from build123d import *

# Parameters (mm, degrees)
PAD005_DEPTH = 9.8
SKETCH007_R  = 6.5
PAD006_DEPTH = 9.8
PAD004_DEPTH = 9.8


with BuildPart() as pad005:
    # Sketch005 → Pad005 (new body)
    with BuildSketch(Plane.XZ.offset(-5)):
        with BuildLine():
            ThreePointArc((42.504006, 47.762261), (40.661796, 52.159127), (36.195109, 53.824922))
            ThreePointArc((23.79127, 66.581039), (27.163695, 57.451626), (36.195109, 53.824922))
            Line((23.79127, 66.581039), (23.79127, 71.581039))
            Line((23.79127, 71.581039), (29.771593, 65.581039))
            ThreePointArc((29.771593, 65.581039), (31.67487, 61.429233), (35.949268, 59.820052))
            ThreePointArc((48.456565, 46.762261), (45.170408, 56.133543), (35.949268, 59.820052))
            Line((48.456565, 46.762261), (48.456565, 41.762261))
            Line((42.504006, 47.762261), (48.456565, 41.762261))
        make_face()
    extrude(amount=PAD005_DEPTH)


with BuildPart() as pad006:
    # Sketch007 → Pad006 (new body)
    with BuildSketch(Plane.XZ.offset(-5)):
        with BuildLine():
            ThreePointArc((24.152058, 13.228672), (35.541387, 1.101686), (47.657351, 12.502741))
            Line((47.657351, 12.502741), (47.657351, 23.35503))
            ThreePointArc((24.152058, 34.470427), (33.144992, 23.076874), (47.657351, 23.35503))
            Line((24.152058, 34.470427), (24.152058, 13.228672))
        make_face()
        with Locations((35.165497, 10.640262)):
            Circle(SKETCH007_R, mode=Mode.SUBTRACT)
    extrude(amount=PAD006_DEPTH)


with BuildPart() as fusion:
    # Sketch006 → Pad004 (new body)
    with BuildSketch(Plane.XZ.offset(-5)):
        with BuildLine():
            Line((33.220749, 59.511791), (33.220749, 28.190693))
            ThreePointArc((33.220749, 28.190693), (46.642574, 22.285891), (47.96319, 36.889591))
            Line((42.96319, 33.791788), (47.96319, 36.889591))
            ThreePointArc((38.220749, 29.859131), (44.504272, 27.107563), (42.96319, 33.791788))
            Line((38.220749, 59.318303), (38.220749, 29.859131))
            Line((33.220749, 59.511791), (38.220749, 59.318303))
        make_face()
    extrude(amount=PAD004_DEPTH)

    # Fusion: union Pad005, Pad006
    add(pad005.part)
    add(pad006.part)


solid = fusion.part
The model under review builds one solid part; all positions refer to its coordinate system, in mm. A direction names the side the tool comes from. Round coordinates to 2 decimals unless told otherwise and drop trailing zeros. Write each loop counter-clockwise with the first axis right and the second up, starting at its lowest first coordinate (ties: lowest second). Pieces come first, ordered by that corner, then holes. Notation, with made-up numbers: (47.5, 55) -> (79.5, 55) arc R33 ccw to (79.5, 90) -> close; hole circle Ø3 at (17, 32). An arc over 180 degrees is marked (long way). Answer as a JSON object with one key per item and string values.
1. We need section A-A on z = 35.5. State the section outline as (x, y) points, and give its area (3 significant figures).
Results found:
{"outline": "(33.22, -4.8) -> (38.22, -4.8) -> (38.22, 5) -> (33.22, 5) -> close; (45.72, -4.8) -> (49.26, -4.8) -> (49.26, 5) -> (45.72, 5) -> close", "area": "83.7 mm^2"}
2. Machinability: for faces 1 (the face through (24.152, 0, 24)), 2 (the face through (48.457, 0, 44)), 3 (the face through (47.657, 0, 18)), 4 (the face through (45.4, 0.2, 35.3)), which of the approach directions +Z, -Z, +X, -X, +Y, -Y give a long, thin tool a straight path to every point of the face, cutting with its end or side? Answer none if there is none.
Results found:
{"face 1": "-Z, -X, +Y, -Y", "face 2": "+X, +Y, -Y", "face 3": "-Z, +X, +Y, -Y", "face 4": "+Y, -Y"}
3. To check wall thickness, follow line 1 along Z through (x, y) = (40.75, 4.5); line 2 along Z through (x, y) = (43.75, 3); line 3 along X through (y, z) = (1, 48). State the ranges of each line that lie inside material, in increasing order.
Results found:
{"line 1": "z = 2.14 to 7.31, 13.97 to 26.45, 52.07 to 59.06", "line 2": "z = 4.1 to 26.62, 33.51 to 34.28, 46.51 to 57.4", "line 3": "x = 33.22 to 38.22, 42.5 to 48.5"}
4. The part is to be moulded in two halves that separate along X. For faces 5 (the face through (37, 5, 29)), 6 (the face through (26.12, 0.17, 58.68)), 7 (the face through (38.221, 0, 42)), say which applies: pulls with the +X half, pulls with the -X half, needs draft (parallel to the pull), parting line crosses it, or undercut.
Results found:
{"face 5": "needs draft", "face 6": "pulls with the -X half", "face 7": "undercut"}
5. We need section C-C on y = 3.5. State the section outline as (x, z) points, and give its area (3 significant figures).
Results found:
{"outline": "(23.79, 66.58) arc R12 ccw to (33.22, 54.09) -> (33.22, 28.19) arc R9.03 ccw to (39.06, 21.55) arc R16.32 cw to (24.15, 34.47) -> (24.15, 13.23) arc R11.76 ccw to (47.66, 12.5) -> (47.66, 22.98) arc R9.03 ccw to (47.96, 36.89) -> (42.96, 33.79) arc R3.84 cw (long way) to (38.22, 29.86) -> (38.22, 53.58) arc R6 cw to (42.5, 47.76) -> (48.46, 41.76) -> (48.46, 46.76) arc R12 ccw to (35.95, 59.82) arc R6 cw to (29.77, 65.58) -> (23.79, 71.58) -> close; hole circle Ø13 at (35.17, 10.64)", "area": "806 mm^2"}
6. We need section D-D on x = 26.25. State the section outline as (y, z) points.
Results found:
{"outline": "(-4.8, 6.14) -> (5, 6.14) -> (5, 29.23) -> (-4.8, 29.23) -> close; (-4.8, 58.51) -> (5, 58.51) -> (5, 69.11) -> (-4.8, 69.11) -> close"}
7. Clearance check with flat-ended pins moving along their axes: pin 1 (1.5 mm diameter, centred on x = 31.5, y = 0.5, fed in from +Z); pin 2 (3 mm diameter, centred on y = -2, z = 39, fed in from -X); pin 3 (4 mm diameter, centred on y = 0.5, z = 16.5, fed in from -X). State where each tip first meets the part, or that it passes through.
Results found:
{"pin 1": "stops at z = 62.53", "pin 2": "stops at x = 33.22", "pin 3": "stops at x = 24.15"}
8. We need section B-B on x = 44.75. State the section outline as (y, z) points, and give its area (3 significant figures).
Results found:
{"outline": "(-4.8, 5.11) -> (5, 5.11) -> (5, 27.33) -> (-4.8, 27.33) -> close; (-4.8, 32.79) -> (5, 32.79) -> (5, 34.9) -> (-4.8, 34.9) -> close; (-4.8, 45.5) -> (5, 45.5) -> (5, 56.55) -> (-4.8, 56.55) -> close", "area": "347 mm^2"}
